Build history of the part. All positions in model axes, mm. A direction names the side the tool comes from. Round coordinates to 2 decimals unless told otherwise and drop trailing zeros. Loops run counter-clockwise (first coordinate to the right, second up) from the corner with the lowest first, then second, coordinate; pieces in that order, holes last. Notation, with made-up numbers: (25, 2) -> (82, 2) arc R23 ccw to (82, 26) -> close; hole circle Ø8 at (68.25, 71). An arc over 180 degrees is marked (long way). Put each result on its own line as item: value. Start each with the question number.
```python
from build123d import *

# Parameters (mm, degrees)
SKETCH1_W           = 67.3
SKETCH1_H           = 40
SKETCH1_R           = 1.65
BOSS_EXTRUDE1_DEPTH = 1.65
SKETCH2_W           = 55.2
SKETCH2_H           = 40
BOSS_EXTRUDE2_DEPTH = 2.5
SKETCH3_W           = 48
SKETCH3_H           = 36.4
CUT_EXTRUDE1_DEPTH  = 0.1


with BuildPart() as part:
    # Sketch1 → Boss-Extrude1 (new body)
    with BuildSketch(Plane(origin=(0, 0, 0), x_dir=(1, 0, 0), z_dir=(0, 1, 0))):
        Rectangle(SKETCH1_W, SKETCH1_H)
        with Locations(Location((-30.7, 17.1, 0), (0, 0, 270))):  # turned: the seam where the file's is
            Circle(SKETCH1_R, mode=Mode.SUBTRACT)
        with Locations(Location((-30.7, -16.75, 0), (0, 0, 270))):  # turned: the seam where the file's is
            Circle(SKETCH1_R, mode=Mode.SUBTRACT)
        with Locations(Location((30.4, -16.75, 0), (0, 0, 270))):  # turned: the seam where the file's is
            Circle(SKETCH1_R, mode=Mode.SUBTRACT)
        with Locations(Location((30.4, 17.1, 0), (0, 0, 270))):  # turned: the seam where the file's is
            Circle(SKETCH1_R, mode=Mode.SUBTRACT)
    extrude(amount=BOSS_EXTRUDE1_DEPTH)

    # Sketch2 → Boss-Extrude2 (add)
    with BuildSketch(Plane(origin=(0, 1.65, 0), x_dir=(1, 0, 0), z_dir=(0, 1, 0))):
        with Locations((0.35, 0)):
            Rectangle(SKETCH2_W, SKETCH2_H)
    extrude(amount=BOSS_EXTRUDE2_DEPTH)

    # Sketch3 → Cut-Extrude1 (cut)
    with BuildSketch(Plane(origin=(0, 4.15, 0), x_dir=(1, 0, 0), z_dir=(0, 1, 0))):
        with Locations((2.05, 0)):
            Rectangle(SKETCH3_W, SKETCH3_H)
    extrude(amount=-CUT_EXTRUDE1_DEPTH, mode=Mode.SUBTRACT)


solid = part.part
```
Item 1: Drop flat-ended pins along their axis: pin 1 (4 mm diameter, centred on x = 30.4, z = 16.75, fed in from -Y); pin 2 (3 mm diameter, centred on x = -29, z = 1.5, fed in from +Y); pin 3 (1.3 mm diameter, centred on y = 2.5, z = 0.5, fed in from +X); pin 4 (0.8 mm diameter, centred on y = 3.5, z = 0, fed in from -X). Give the stop position or say it passes through.
Item 2: Pull direction X, two halves, no side cores. Call faces 1 (the face through (31.79, 0.81, -16.21)), 2 (the face through (-30, 1.65, 0)), 3 (the face through (-27.25, 3, 0)): +X half, -X half, draft (parallel to the pull), parting line (faces both ways), or undercut.
Item 3: Cut at B-B on z = 16.75. Write the cut outline in (x, y), then the cut area to 3 significant figures.
Item 4: Cut at C-C on z = -14.5. Write the cut outline in (x, y).
Item 5: Cut at A-A on x = 30.4. Write the cut outline in (y, z).
Item 6: Wall check: line 1 (X direction, y = 0.55, z = 16.75); line 2 (Y direction, x = 14, z = 16.5); line 3 (X direction, y = 0.8, z = -18). Give the ranges that are in metal, low to high. Write a range as from..to.
Item 7: 3-axis set-ups, long thin cutter, end or side, ignore diameter. For faces 4 (the face through (0, 0, 0)), 5 (the face through (2, 4.05, 0)), 6 (the face through (27.95, 3, 0)): which of +Z, -Z, +X, -X, +Y, -Y reach the whole face in a straight line?
Item 8: Cut at D-D on x = 10. Write the cut outline in (y, z), then the cut area to 3 significant figures.
Ans:
1. pin 1: stops at y = 0
1. pin 2: stops at y = 1.65
1. pin 3: stops at x = 27.95
1. pin 4: stops at x = -27.25
2. face 1: undercut
2. face 2: draft
2. face 3: -X half
3. outline: (-33.65, 0) -> (-32.35, 0) -> (-32.35, 1.65) -> (-33.65, 1.65) -> close; (-29.05, 0) -> (28.75, 0) -> (28.75, 1.65) -> (27.95, 1.65) -> (27.95, 4.15) -> (26.05, 4.15) -> (26.05, 4.05) -> (-21.95, 4.05) -> (-21.95, 4.15) -> (-27.25, 4.15) -> (-27.25, 1.65) -> (-29.05, 1.65) -> close; (32.05, 0) -> (33.65, 0) -> (33.65, 1.65) -> (32.05, 1.65) -> close
3. area: 233 mm2
4. outline: (-33.65, 0) -> (33.65, 0) -> (33.65, 1.65) -> (27.95, 1.65) -> (27.95, 4.15) -> (26.05, 4.15) -> (26.05, 4.05) -> (-21.95, 4.05) -> (-21.95, 4.15) -> (-27.25, 4.15) -> (-27.25, 1.65) -> (-33.65, 1.65) -> close
5. outline: (0, -20) -> (1.65, -20) -> (1.65, -18.75) -> (0, -18.75) -> close; (0, -15.45) -> (1.65, -15.45) -> (1.65, 15.1) -> (0, 15.1) -> close; (0, 18.4) -> (1.65, 18.4) -> (1.65, 20) -> (0, 20) -> close
6. line 1: x = -33.65..-32.35, -29.05..28.75, 32.05..33.65
6. line 2: y = 0..4.05
6. line 3: x = -33.65..-32.08, -29.32..29.02, 31.78..33.65
7. face 4: +Z, -Z, +X, -X, -Y
7. face 5: +Y
7. face 6: +Z, -Z, +X, +Y
8. outline: (0, -20) -> (4.15, -20) -> (4.15, -18.2) -> (4.05, -18.2) -> (4.05, 18.2) -> (4.15, 18.2) -> (4.15, 20) -> (0, 20) -> close
8. area: 162 mm2
